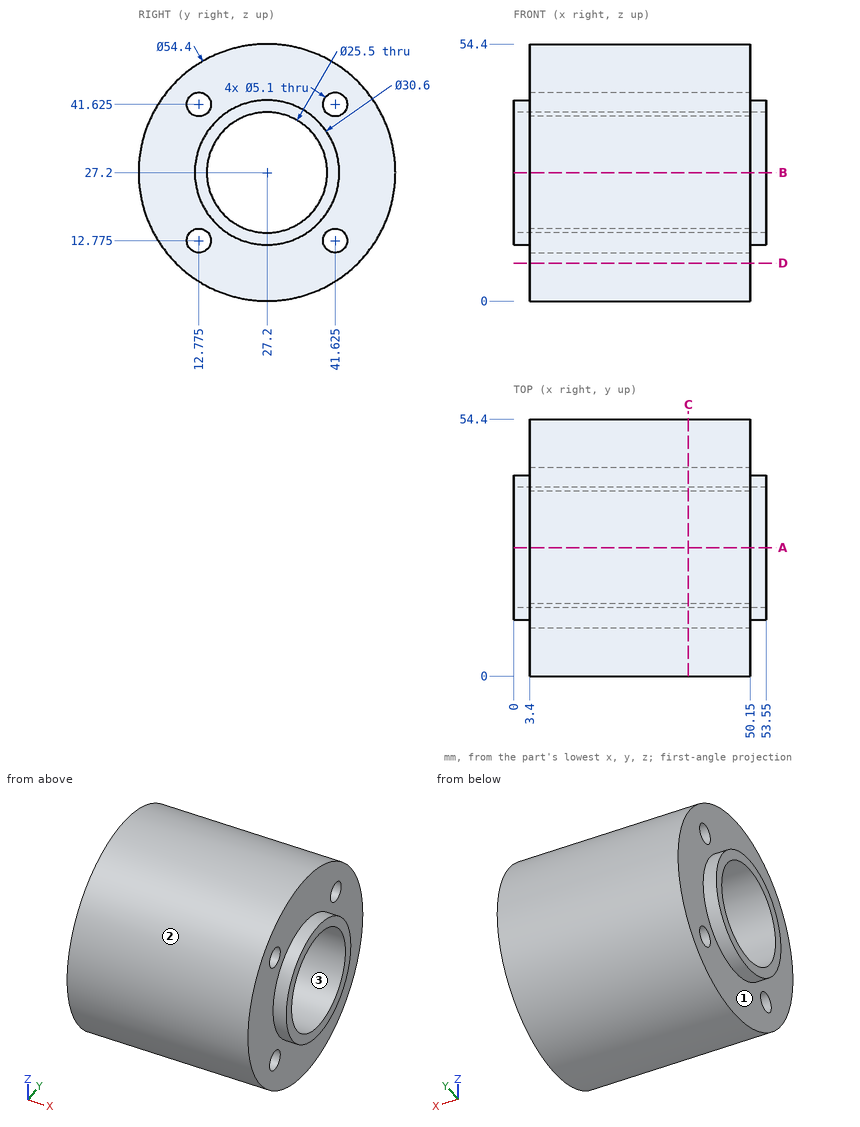
For this review, use the dimensioned drawing (mm, ordinates from the lowest corner) and the shaded views. Coordinates: 2 decimals unless noted, no trailing zeros. Loops run counter-clockwise (first coordinate to the right, second up) from the corner with the lowest first, then second, coordinate; pieces in that order, holes last. Notation, with made-up numbers: (49, 49) -> (74, 49) arc R34 ccw to (74, 79) -> close; hole circle Ø11 at (72, 73). An arc over 180 degrees is marked (long way). Use a Markdown table: item, result. Add a question column.
1. To check wall thickness, follow line 1 (Z direction, x = 7, y = 40); line 2 (Z direction, x = 22, y = 27); line 3 (Y direction, x = 50.5, z = 27). State the ranges of each line that lie inside material, in increasing order.
2. Draft analysis for pull direction Z (two halves, no side actions). For the marked faces 1, 2 and 3, state which applies: pulls with the +Z half, pulls with the -Z half, needs draft (parallel to the pull), parting line crosses it, or undercut.
3. Add section A-A on y = 27.2. Write out the cut boundary in (x, z).
4. Add section C-C on x = 37. Write out the cut boundary in (y, z) (3 decimals), plus the area to 3 significant figures.
5. Add section D-D on z = 8. Write out the cut boundary in (x, y).
6. Clearance check with flat-ended pins moving along their axes: pin 1 Ø1.5 at (y, z) = (6, 22) entering from -X; pin 2 Ø8 at (x, z) = (42, 8.5) entering from -Y; pin 3 Ø10 at (x, y) = (13.5, 26.5) entering from -Z. State where each tip first meets the part, or that it passes through.
Returned:
| question | item | result |
|---|---|---|
| 1 | line 1 | z = 3.2 to 10.81, 14.74 to 39.66, 43.59 to 51.2 |
| 1 | line 2 | z = 0 to 14.45, 39.95 to 54.4 |
| 1 | line 3 | y = 11.9 to 14.45, 39.95 to 42.5 |
| 2 | face 1 | needs draft |
| 2 | face 2 | parting line crosses it |
| 2 | face 3 | undercut |
| 3 | outline | (0, 11.9) -> (3.4, 11.9) -> (3.4, 0) -> (50.15, 0) -> (50.15, 11.9) -> (53.55, 11.9) -> (53.55, 14.45) -> (0, 14.45) -> close; (0, 39.95) -> (53.55, 39.95) -> (53.55, 42.5) -> (50.15, 42.5) -> (50.15, 54.4) -> (3.4, 54.4) -> (3.4, 42.5) -> (0, 42.5) -> close |
| 4 | outline | circle Ø54.4 at (27.2, 27.2); hole circle Ø5.1 at (12.775, 12.775); hole circle Ø5.1 at (12.775, 41.625); hole circle Ø25.5 at (27.2, 27.2); hole circle Ø5.1 at (41.625, 12.775); hole circle Ø5.1 at (41.625, 41.625) |
| 4 | area | 1,730 mm² |
| 5 | outline | (3.4, 7.93) -> (50.15, 7.93) -> (50.15, 46.47) -> (3.4, 46.47) -> close |
| 6 | pin 1 | stops at x = 3.4 |
| 6 | pin 2 | stops at y = 4.31 |
| 6 | pin 3 | stops at z = 0 |
